Geometry: final body of the model. Coordinates: model frame, mm. Give positions to 0.01 mm unless a question says otherwise; leave off trailing zeros. Order: outer loops, then holes, each group sorted by start corner. A loop starts at its lowest first (then second) coordinate and runs counter-clockwise, first axis right, second up. Notation, with made-up numbers: (50.5, 65) -> (103.5, 65) arc R25 ccw to (103.5, 97) -> close; hole circle Ø7 at (55, 41.5). An arc over 180 degrees is marked (long way). Answer in a Markdown table with one row per item. Add a question column.
Q1. Line query: line 1 along X through (y, z) = (38.5, 2.5); line 2 along X through (y, z) = (35, 2.35); line 3 along X through (y, z) = (21, 4.3). Output: solid intervals per line, ascending. Write a range as from..to.
Q2. Cut plane B-B on x = 34. Return the cut outline in (y, z), and give its area (3 significant figures).
Q3. Cut plane A-A on y = 23. Return the cut outline in (x, z).
Q4. Contact query for flat-ended pins moving along their axis: P1, Ø1.5, axis at x = 53.5, z = 3.5, coming from the -Y side; P2, Ø0.6, axis at x = 24, z = 2.5, coming from the -Y side; P3, Ø1.5, axis at y = 40.5, z = 2.5, coming from the -X side. Output: stop coordinate, or through.
Q5. Cut plane C-C on x = -25. Return the cut outline in (y, z).
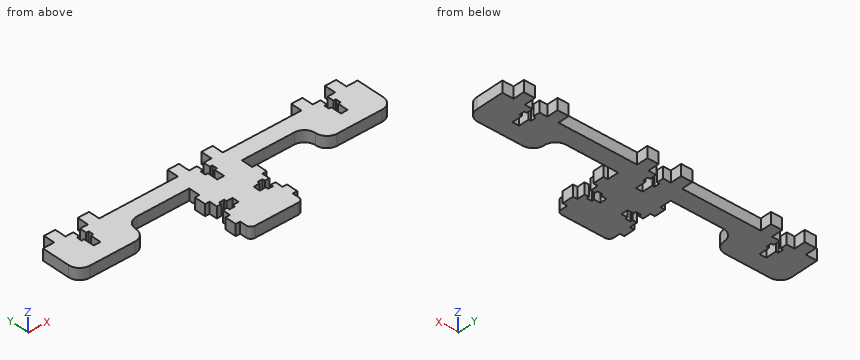
from build123d import *

# Parameters (mm, degrees)
BOSS_EXTRU_1_DEPTH = 5
CONG_1_R           = 5
FILLET1_R          = 2


with BuildPart() as part:
    # Esquisse1 → Boss.-Extru.1 (new body)
    with BuildSketch(Plane.XY):
        Polygon((25.4, 25), (23.4, 25), (23.4, 30), (51.7, 30), (51.7, 20), (81.7, 20), (81.7, 37.5), (76.7, 37.5), (76.7, 42.5), (71.7, 42.5), (71.7, 37.5), (68.2, 37.5), (68.2, 34.5), (69.3, 34.5), (69.3, 32.2), (68.2, 32.2), (68.2, 27.5), (65.2, 27.5), (65.2, 32.2), (64.1, 32.2), (64.1, 34.5), (65.2, 34.5), (65.2, 37.5), (61.7, 37.5), (61.7, 42.5), (56.7, 42.5), (56.7, 37.5), (21.7, 37.5), (21.7, 42.5), (16.7, 42.5), (16.7, 37.5), (13.2, 37.5), (13.2, 34.5), (14.3, 34.5), (14.3, 32.2), (13.2, 32.2), (13.2, 27.5), (10.2, 27.5), (10.2, 32.2), (9.1, 32.2), (9.1, 34.5), (10.2, 34.5), (10.2, 37.5), (6.7, 37.5), (6.7, 42.5), (1.7, 42.5), (1.7, 37.5), (-33.3, 37.5), (-33.3, 42.5), (-38.3, 42.5), (-38.3, 37.5), (-41.8, 37.5), (-41.8, 34.5), (-40.7, 34.5), (-40.7, 32.2), (-41.8, 32.2), (-41.8, 27.5), (-44.8, 27.5), (-44.8, 32.2), (-45.9, 32.2), (-45.9, 34.5), (-44.8, 34.5), (-44.8, 37.5), (-48.3, 37.5), (-48.3, 42.5), (-53.3, 42.5), (-53.3, 37.5), (-58.3, 37.5), (-58.3, 20), (-28.3, 20), (-28.3, 30), (0, 30), (0, 25), (-2, 25), (-2, 20), (0, 20), (0, 16.5), (2, 16.5), (2, 17.6), (4.3, 17.6), (4.3, 16.5), (7, 16.5), (7, 13.5), (4.3, 13.5), (4.3, 12.4), (2, 12.4), (2, 13.5), (0, 13.5), (0, 10), (-2, 10), (-2, 5), (0, 5), (0, 0), (23.4, 0), (23.4, 5), (25.4, 5), (25.4, 10), (23.4, 10), (23.4, 13.5), (21.4, 13.5), (21.4, 12.4), (19.1, 12.4), (19.1, 13.5), (16.4, 13.5), (16.4, 16.5), (19.1, 16.5), (19.1, 17.6), (21.4, 17.6), (21.4, 16.5), (23.4, 16.5), (23.4, 20), (25.4, 20), align=None)
    extrude(amount=BOSS_EXTRU_1_DEPTH)

    # Congé1
    cong_1_edges = [part.edges().sort_by_distance(p)[0] for p in [
        (-28.3, 30, 2.5),
        (-58.3, 20, 2.5),
        (-28.3, 20, 2.5),
        (81.7, 20, 2.5),
        (51.7, 20, 2.5),
        (51.7, 30, 2.5),
    ]]
    fillet(cong_1_edges, radius=CONG_1_R - 0.0001)  # a hair under: the kernel refuses the full size

    # Fillet1
    fillet1_edges = [part.edges().sort_by_distance(p)[0] for p in [
        (23.4, 0, 2.5),
        (0, 0, 2.5),
    ]]
    fillet(fillet1_edges, radius=FILLET1_R)


solid = part.part
Completed:
| question | item | result |
|---|---|---|
| 1 | line 1 | x = -53.3..-48.3, -38.3..-33.3, 1.7..6.7, 16.7..21.7, 56.7..61.7, 71.7..76.7 |
| 1 | line 2 | x = -58.3..-44.8, -41.8..10.2, 13.2..65.2, 68.2..81.7 |
| 1 | line 3 | x = -56.3..-30.3, -2..25.4, 53.7..79.7 |
| 2 | outline | (30, 0) -> (37.5, 0) -> (37.5, 5) -> (30, 5) -> close |
| 2 | area | 37.5 mm² |
| 3 | outline | (-57.88, 0) -> (-28.72, 0) -> (-28.72, 5) -> (-57.88, 5) -> close; (-2, 0) -> (25.4, 0) -> (25.4, 5) -> (-2, 5) -> close; (52.12, 0) -> (81.28, 0) -> (81.28, 5) -> (52.12, 5) -> close |
| 4 | P1 | stops at y = 20.64 |
| 4 | P2 | stops at y = 5 |
| 4 | P3 | stops at x = -53.3 |
| 5 | outline | (29.7, 0) -> (37.5, 0) -> (37.5, 5) -> (29.7, 5) -> close |
